Geometry: final body of the model. Coordinates: model frame, mm. Face numbers are marked on the shaded views. Give positions to 0.01 mm unless a question says otherwise; leave off trailing zeros. Write each loop counter-clockwise with the first axis right and the second up, starting at its lowest first coordinate (ties: lowest second). Pieces come first, ordered by that corner, then holes.
Q1. Draft query along Z for the marked faces 1, 2, 3 and 4. Return one class per face: pulls with the +Z half, pulls with the -Z half, needs draft (parallel to the pull), parting line crosses it, or undercut.
Q2. Line query: L1, parallel to Y at x = 11.5, z = 9.5; L2, parallel to Y at x = -15, z = 7.75. Output: solid intervals per line, ascending.
Q3. Cut plane A-A on z = 8.25. Return the cut outline in (x, y).
Q4. Cut plane B-B on x = -14. Return the cut outline in (y, z), plus the area to 3 significant figures.
```python
from build123d import *

# Parameters (mm, degrees)
SKETCH1_W           = 60
SKETCH1_H           = 25
BOSS_EXTRUDE1_DEPTH = 19.8
CUT_EXTRUDE3_DEPTH  = 19.8
BOSS_EXTRUDE2_DEPTH = 1
BOSS_EXTRUDE3_START = -18.8
BOSS_EXTRUDE3_DEPTH = 1


with BuildPart() as part:
    # Sketch1 → Boss-Extrude1 (new body)
    with BuildSketch(Plane.XY):
        with Locations((0, 12.5)):
            Rectangle(SKETCH1_W, SKETCH1_H)
    extrude(amount=BOSS_EXTRUDE1_DEPTH)

    # Sketch2 → Cut-Extrude3 (cut)
    with BuildSketch(Plane(origin=(0, 0, 0), x_dir=(-1, 0, 0), z_dir=(0, 0, -1))):
        with BuildLine():
            Line((-20, 0), (-8, 0))
            ThreePointArc((-8, 0), (-14, 6), (-20, 0))
        make_face()
        with BuildLine():
            Line((8, 0), (20, 0))
            ThreePointArc((20, 0), (14, 6), (8, 0))
        make_face()
    extrude(amount=-CUT_EXTRUDE3_DEPTH, mode=Mode.SUBTRACT)

    # Sketch4 → Boss-Extrude2 (add)
    with BuildSketch(Plane(origin=(0, 0, 0), x_dir=(-1, 0, 0), z_dir=(0, 0, -1))):
        with BuildLine():
            Line((-19.75, 0), (-20, 0))
            ThreePointArc((-20, 0), (-14, 6), (-8, 0))
            Line((-8, 0), (-8.25, 0))
            ThreePointArc((-8.25, 0), (-14, 5.75), (-19.75, 0))
        make_face()
        with BuildLine():
            Line((8, 0), (8.25, 0))
            ThreePointArc((8.25, 0), (14, 5.75), (19.75, 0))
            Line((19.75, 0), (20, 0))
            ThreePointArc((20, 0), (14, 6), (8, 0))
        make_face()
    extrude(amount=-BOSS_EXTRUDE2_DEPTH)

    # Sketch4<2> → Boss-Extrude3 (add)
    with BuildSketch(Plane(origin=(0, 0, 0), x_dir=(-1, 0, 0), z_dir=(0, 0, -1)).offset(BOSS_EXTRUDE3_START)):
        with BuildLine():
            Line((-19.75, 0), (-20, 0))
            ThreePointArc((-20, 0), (-14, 6), (-8, 0))
            Line((-8, 0), (-8.25, 0))
            ThreePointArc((-8.25, 0), (-14, 5.75), (-19.75, 0))
        make_face()
        with BuildLine():
            Line((8, 0), (8.25, 0))
            ThreePointArc((8.25, 0), (14, 5.75), (19.75, 0))
            Line((19.75, 0), (20, 0))
            ThreePointArc((20, 0), (14, 6), (8, 0))
        make_face()
    extrude(amount=-BOSS_EXTRUDE3_DEPTH)


solid = part.part
```
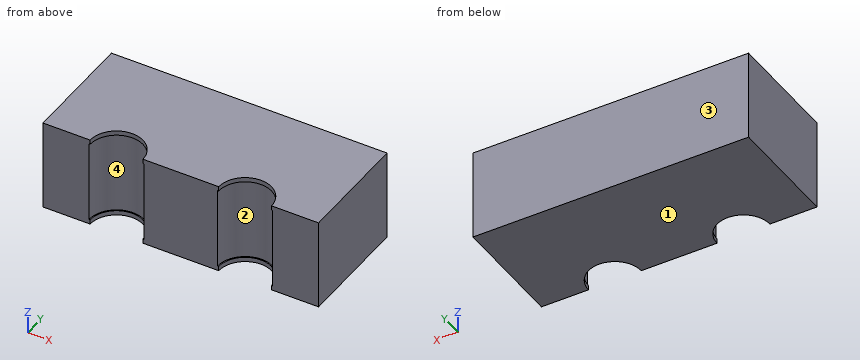
Data:
1. face 1: pulls with the -Z half
1. face 2: undercut
1. face 3: needs draft
1. face 4: undercut
2. L1: y = 5.45 to 25
2. L2: y = 5.92 to 25
3. outline: (-30, 0) - (-20, 0) arc R6 cw to (-8, 0) - (8, 0) arc R6 cw to (20, 0) - (30, 0) - (30, 25) - (-30, 25) - close
4. outline: (5.75, 0) - (25, 0) - (25, 19.8) - (5.75, 19.8) - (5.75, 18.8) - (6, 18.8) - (6, 1) - (5.75, 1) - close
4. area: 377 mm2
